Here's how the part is built. I have some questions about the finished solid (model axes, mm). A direction names the side the tool comes from. Coordinates: 2 decimals unless noted, no trailing zeros. Write each loop counter-clockwise with the first axis right and the second up, starting at its lowest first coordinate (ties: lowest second). Pieces come first, ordered by that corner, then holes.
(1) Imagine slicing it at B-B, the plane z = 38.1. List the corners of the cut face in (x, y) for me (3 decimals), plus the area to 3 significant figures.
(2) Thinking about a two-plate mould opening in Y: for faces 5 (the flat face through (70, 41.275, 51)), 6 (the cylindrical face through (69.939, 14.991, -48.627)), 7 (the flat face through (70, 88.9, 52)), which applies, released by +Y, released by -Y, zero draft, split by the parting line, or undercut?
(3) Imagine slicing it at A-A, the plane y = 50.8. List the corners of the cut face in (x, z) for me (3 decimals), plus the area to 3 significant figures.
(4) Imagine slicing it at C-C, the plane z = 16. List the corners of the cut face in (x, y) for me, plus the area to 3 significant figures.
(5) Which directions (+Z, -Z, +X, -X, +Y, -Y) give clear straight access to the entire face, cutting with the end or side of a thin tool? Please do faces 1 (the flat face through (32, 6, 104.521)), 2 (the flat face through (63.5, 34, 52)), 3 (the flat face through (70, 12.7, -21)), 4 (the cylindrical face through (69.761, 51.009, 25.402)).
(6) For pin 1 Ø19 at (x, z) = (37, 109) entering from +Y; pin 2 Ø4 at (x, y) = (33.5, 4.5) entering from -Z; pin 3 Ø4 at (x, z) = (68, -29) entering from -Y, each with a flat end and sliding along its axis, tell me the tip position at first contact or that it passes through.
(7) Imagine slicing it at D-D, the plane z = 107.5. List the corners of the cut face in (x, y) for me, plus the area to 3 significant figures.
(8) Please list where these lines run through material, in increasing order: probe 1 along Z at (x, y) = (70.25, 50.8) (3 decimals); probe 2 along Z at (x, y) = (71, 50); probe 3 along Y at (x, z) = (70.5, 50) (3 decimals).
```python
from build123d import *

# Parameters (mm, degrees)
F1_DEPTH  = 152.146
F2_W      = 12.7
F2_H      = 76.2
F3_DEPTH  = 50.8
F4_R      = 7.62
F5_R      = 7.62
F6_R      = 7.62
F8_DEPTH  = 25.4
F9_R      = 9.525
F10_DEPTH = 12.701


with BuildPart() as f1:
    # F0 (on Top) → F1 (new body)
    with BuildSketch(Plane.XY):
        Polygon((0, 12.7), (0, 0), (76.2, 0), (76.2, 88.9), (63.5, 88.9), (63.5, 12.7), align=None)
    extrude(amount=F1_DEPTH)

    # F2 (on face) → F3 (join)
    with BuildSketch(Plane(origin=(0, 0, 0), x_dir=(1, 0, 0), z_dir=(0, 0, -1))):
        with Locations((69.85, -50.8)):
            Rectangle(F2_W, F2_H)
    extrude(amount=F3_DEPTH)

    # F4
    f4_edges = [f1.edges().sort_by_distance(p)[0] for p in [
        (0, 6.35, 0),
        (0, 6.35, 152.146),
    ]]
    fillet(f4_edges, radius=F4_R)

    # F5
    f5_edges = [f1.edges().sort_by_distance(p)[0] for p in [
        (69.85, 88.9, 152.146),
    ]]
    fillet(f5_edges, radius=F5_R)

    # F6
    f6_edges = [f1.edges().sort_by_distance(p)[0] for p in [
        (69.85, 12.7, -50.8),
        (69.85, 88.9, -50.8),
    ]]
    fillet(f6_edges, radius=F6_R)

    # F7 (on face) → F8 (cut)
    with BuildSketch(Plane(origin=(0, 12.7, 0), x_dir=(-1, 0, 0), z_dir=(0, 1, 0))):
        with BuildLine():
            Line((-46.99, 28.575), (-16.51, 28.575))
            ThreePointArc((-16.51, 28.575), (-6.985, 38.1), (-16.51, 47.625))
            Line((-16.51, 47.625), (-46.99, 47.625))
            ThreePointArc((-46.99, 47.625), (-56.515, 38.1), (-46.99, 28.575))
        make_face()
        with BuildLine():
            Line((-46.99, 104.521), (-16.51, 104.521))
            ThreePointArc((-16.51, 104.521), (-6.985, 114.046), (-16.51, 123.571))
            Line((-16.51, 123.571), (-46.99, 123.571))
            ThreePointArc((-46.99, 123.571), (-56.515, 114.046), (-46.99, 104.521))
        make_face()
    extrude(amount=-F8_DEPTH, mode=Mode.SUBTRACT)

    # F9 (on face) → F10 (cut, through all)
    with BuildSketch(Plane(origin=(63.5, 0, 0), x_dir=(0, -1, 0), z_dir=(-1, 0, 0))):
        with Locations((-50.8, -25.4)):
            Circle(F9_R)
        with BuildLine():
            Line((-41.275, 34.925002), (-41.275, 66.675002))
            ThreePointArc((-41.275, 66.675002), (-50.800002, 76.199998), (-60.325, 66.674998))
            Line((-60.325, 66.674998), (-60.325, 34.924998))
            ThreePointArc((-60.325, 34.924998), (-50.799998, 25.399998), (-41.275, 34.925002))
        make_face()
        with Locations((-50.8, 126.746)):
            Circle(F9_R)
    extrude(amount=-F10_DEPTH, mode=Mode.SUBTRACT)


solid = f1.part
```
Recorded:
1. outline: (0, 0) - (6.985, 0) - (6.985, 12.7) - (0, 12.7) - close; (56.515, 0) - (76.2, 0) - (76.2, 41.275) - (63.5, 41.275) - (63.5, 12.7) - (56.515, 12.7) - close; (63.5, 60.325) - (76.2, 60.325) - (76.2, 88.9) - (63.5, 88.9) - close
1. area: 1,060 mm2
2. face 5: undercut
2. face 6: released by -Y
2. face 7: released by +Y
3. outline: (63.5, -50.8) - (76.2, -50.8) - (76.2, -34.925) - (63.5, -34.925) - close; (63.5, -15.875) - (76.2, -15.875) - (76.2, 25.4) - (63.5, 25.4) - close; (63.5, 76.2) - (76.2, 76.2) - (76.2, 117.221) - (63.5, 117.221) - close; (63.5, 136.271) - (76.2, 136.271) - (76.2, 152.146) - (63.5, 152.146) - close
3. area: 1,450 mm2
4. outline: (0, 0) - (76.2, 0) - (76.2, 88.9) - (63.5, 88.9) - (63.5, 12.7) - (0, 12.7) - close
4. area: 1,940 mm2
5. face 1: +Y, -Y
5. face 2: +Z, -Z, -X, +Y
5. face 3: -Z, +X, -X, -Y
5. face 4: +X, -X
6. pin 1: stops at y = 12.7
6. pin 2: stops at z = 0
6. pin 3: stops at y = 12.7
7. outline: (0, 0) - (9.59, 0) - (9.59, 12.7) - (0, 12.7) - close; (53.91, 0) - (76.2, 0) - (76.2, 88.9) - (63.5, 88.9) - (63.5, 12.7) - (53.91, 12.7) - close
7. area: 1,370 mm2
8. probe 1: z = -50.8 to -34.925, -15.875 to 25.4, 76.2 to 117.221, 136.271 to 152.146
8. probe 2: z = -50.8 to -34.89, -15.91 to 25.43, 76.17 to 117.25, 136.24 to 152.15
8. probe 3: y = 0 to 41.275, 60.325 to 88.9
